Here's how the part is built. I have some questions about the finished solid (model axes, mm). Face numbers are marked on the shaded views. A direction names the side the tool comes from. Give positions to 0.01 mm unless a question says otherwise; leave off trailing zeros. Order: outer loops, then holes, each group sorted by start corner. A loop starts at its lowest first (then second) coordinate and runs counter-clockwise, first axis right, second up. Notation, with made-up numbers: M -22,80.25 L 17,80.25 A15 cw 17,104.25 Z; hole C -37,48 d10. An arc over 180 degrees is marked long. Use CSV: the item, a comma, the result in double quotes. Start each with the question number.
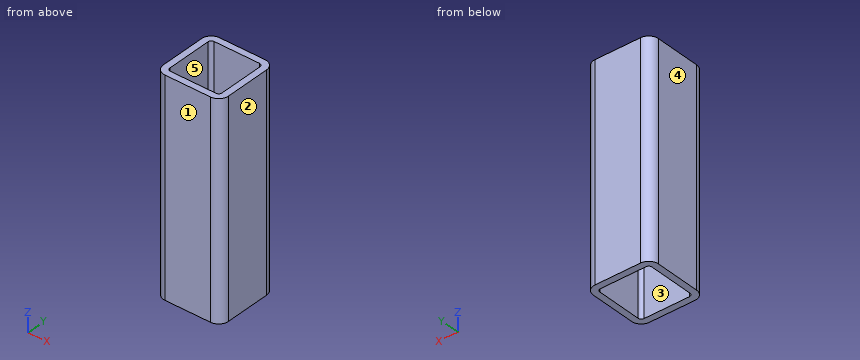
Autodesk Inventor part; units mm, degrees
ref_plane "Start Plane" through (0, 0, 10) normal (0, 0, 1) x (1, 0, 0)
ref_plane "End Plane" through (0, 0, 75) normal (0, 0, 1) x (1, 0, 0)
ref_plane "Work Plane4" through (7, -120, 10) normal (0, 0, -1) x (-1, 0, 0)
ref_plane "Start Plane" through (0, 0, 10) normal (0, 0, 1) x (1, 0, 0)
ref_plane "End Plane" through (0, 0, 75) normal (0, 0, 1) x (1, 0, 0)
sketch "Sketch" plane through (0, 0, 0) normal (0, 0, 1) x (1, 0, 0)
  line L0 (-10, -7) -> (-10, 7)
  line L1 (-7, 10) -> (7, 10)
  line L2 (10, 7) -> (10, -7)
  line L3 (7, -10) -> (-7, -10)
  arc A0 (-10, -7) -> (-7, -10) centre (-7, -7) ccw
  arc A1 (-7, 10) -> (-10, 7) centre (-7, 7) ccw
  arc A2 (10, 7) -> (7, 10) centre (7, 7) ccw
  arc A3 (7, -10) -> (10, -7) centre (7, -7) ccw
  arc A4 (-7, 8) -> (-8, 7) centre (-7, 7) ccw
  line L4 (-7, 8) -> (7, 8)
  arc A5 (8, 7) -> (7, 8) centre (7, 7) ccw
  line L5 (8, 7) -> (8, -7)
  arc A6 (7, -8) -> (8, -7) centre (7, -7) ccw
  line L6 (7, -8) -> (-7, -8)
  arc A7 (-8, -7) -> (-7, -8) centre (-7, -7) ccw
  line L7 (-8, -7) -> (-8, 7)
  line L8 (0, 14.8698) -> (0, -14.8698) construction
  line L9 (-14.8698, 0) -> (14.8698, 0) construction
  dimension "d7" = 3
  dimension "d10" = 20
  dimension "d11" = 20
  dimension "d12" = 2
  dimension "d15" = 10
  dimension "d16" = 10
extrude "Body" add sketch "Sketch" along normal up to surface (65 mm away) from surface at 10
sketch "Sketch3" plane through (0, 0, 0) normal (0, 0, 1) x (1, 0, 0)
  line L0 (0, 0) -> (10, 0)
ref_plane "Work Plane3" through (0, 0, 0) normal (0, -1, 0) x (1, 0, 0)
sketch "Sketch4" plane through (0, 0, 0) normal (0, -1, 0) x (1, 0, 0)
  line L0 (-2, 10) -> (12, 10)
  line L1 (-2, 75) -> (12, 75)
  dimension "d18" = 65
ref_plane "Work Plane4" through (7, -120, 10) normal (0, 0, -1) x (-1, 0, 0)
split "Split1" plane through (7, -120, 10) removes the side toward (0, 0, -1)
equation "\"d7\" = G_IR"
equation "\"d10\" = G_H"
equation "\"d11\" = G_W"
equation "\"d12\" = G_T"
equation "\"d15\" = 0.5 * d10"
equation "\"d16\" = 0.5 * d11"
equation "\"d3\" = G_L"
equation "\"G_W\" = 20"
equation "\"G_H\" = 20"
equation "\"G_T\" = 2"
equation "\"G_IR\" = 3"
equation "\"G_L\" = d18"
equation "\"G_OFFSET_END\" = 0"
equation "\"d14\" = G_OFFSET_END + B_L"
equation "\"B_L\" = 75"
properties part number "ISO 12633-2 - 20x20x2 - 65" material "Steel, Mild"
Q1. I need wall thicknesses on line 1 (X direction, y = -0.5, z = 59); line 2 (Y direction, x = 7.75, z = 37). Which ranges of each line are inside material? Lowest first, please. Write a range as [from, to].
Q2. Imagine slicing it at C-C, the plane z = 50.5. Please give me the cut outline in (x, y).
Q3. Imagine slicing it at A-A, the plane x = 3. Please give me the cut outline in (y, z), then the cut area to 3 significant figures.
Q4. We'd pull the mould along X, two halves only. Please class the marked faces 1, 2 and 3: pulls with the +X half, pulls with the -X half, needs draft (parallel to the pull), parting line crosses it, or undercut.
Q5. For P1, Ø4, axis at x = -7, y = -7, coming from the +Z side, with a flat end and sliding along its axis, tell me the tip position at first contact or that it passes through.
Q6. Imagine slicing it at D-D, the plane y = 8.75. Please give me the cut outline in (x, z).
Q7. For the marked faces 4 and 5, which set-ups out of +Z, -Z, +X, -X, +Y, -Y let a thin tool reach every point of the face, with its end or its side?
Reply:
1,line 1,"x = [-10, -8], [8, 10]"
1,line 2,"y = [-9.9, -7.66], [7.66, 9.9]"
2,outline,"M -10,-7 A3 ccw -7,-10 L 7,-10 A3 ccw 10,-7 L 10,7 A3 ccw 7,10 L -7,10 A3 ccw -10,7 Z; hole M -8,-7 A1 ccw -7,-8 L 7,-8 A1 ccw 8,-7 L 8,7 A1 ccw 7,8 L -7,8 A1 ccw -8,7 Z"
3,outline,"M -10,10 L -8,10 L -8,75 L -10,75 Z; M 8,10 L 10,10 L 10,75 L 8,75 Z"
3,area,"260 mm^2"
4,face 1,"needs draft"
4,face 2,"pulls with the +X half"
4,face 3,"undercut"
5,P1,"stops at z = 75"
6,outline,"M -9.44,10 L 9.44,10 L 9.44,75 L -9.44,75 Z"
7,face 4,"+Z, -Z, -X, +Y, -Y"
7,face 5,"+Z, -Z"
